Part model, mm, in its own coordinate system. A direction names the side the tool comes from. Round coordinates to 2 decimals unless told otherwise and drop trailing zeros. Write each loop counter-clockwise with the first axis right and the second up, starting at its lowest first coordinate (ties: lowest second). Pieces come first, ordered by that corner, then holes.
Autodesk Inventor part; units mm, degrees
ref_plane "YZ Plane" through (0, 0, 0) normal (1, 0, 0) x (0, 1, 0)
ref_plane "XZ Plane" through (0, 0, 0) normal (0, 1, 0) x (-1, 0, 0)
ref_plane "XY Plane" through (0, 0, 0) normal (0, 0, 1) x (1, 0, 0)
sketch "Esboço1" plane through (0, 0, 0) normal (0, 1, 0) x (-1, 0, 0)
  line L0 (5, 0) -> (70, 0)
  line L1 (75, -5) -> (75, -70)
  line L2 (70, -75) -> (5, -75)
  line L3 (0, -70) -> (0, -5)
  arc A0 (70, -75) -> (75, -70) centre (70, -70) ccw
  arc A1 (0, -70) -> (5, -75) centre (5, -70) ccw
  arc A2 (75, -5) -> (70, 0) centre (70, -5) ccw
  arc A3 (5, 0) -> (0, -5) centre (5, -5) ccw
  point P0 (0, 0)
  point P1 (75, -75)
  point P2 (75, 0)
  point P3 (0, -75)
  dimension "d0" = 75
  dimension "d1" = 75
  dimension "d2" = 5
extrude "Extrusão1" add sketch "Esboço1" along normal blind 5
sketch "Esboço2" plane through (0, 5, 0) normal (0, 1, 0) x (1, 0, 0)
  line L0 (0, 75) -> (-13, 75)
  line L1 (-75, 75) -> (-62, 75)
  line L2 (-75, 0) -> (-62, 0)
  line L3 (-70, 0) -> (-5, 0)
  line L4 (0, 0) -> (-13, 0)
  line L5 (-13, 75) -> (-13, 72.5)
  line L6 (-62, 75) -> (-62, 72.5)
  line L7 (-62, 0) -> (-62, 2.5)
  line L8 (-13, 0) -> (-13, 2.5)
  circle A0 centre (-62, 72.5) radius 1.25
  circle A1 centre (-13, 72.5) radius 1.25
  circle A2 centre (-62, 2.5) radius 1.25
  circle A3 centre (-13, 2.5) radius 1.25
  dimension "d5" = 13
  dimension "d6" = 2.5
  dimension "d7" = 2.5
  dimension "d8" = 2.5
  dimension "d9" = 2.5
  dimension "d10" = 2.5
  dimension "d11" = 2.5
extrude "Extrusão2" cut sketch "Esboço2" against normal through all
sketch "Esboço3" plane through (0, 0, 0) normal (0, -1, 0) x (1, 0, 0)
  line L0 (-5, -75) -> (-70, -75)
  line L1 (-5, -75) -> (-5, -70)
  line L2 (-5, -70) -> (-70, -70)
  line L3 (-70, -70) -> (-70, -5)
  line L4 (-70, -5) -> (-5, -5)
  line L5 (-5, -5) -> (-5, -70)
  point P0 (0, 0)
  dimension "d14" = 5
  dimension "d15" = 65
  dimension "d16" = 65
extrude "Extrusão3" cut sketch "Esboço3" against normal blind 2.5
sketch "Esboço4" plane through (0, 5, 0) normal (0, 1, 0) x (1, 0, 0)
  line L0 (-5, 70) -> (-70, 70)
  line L1 (-70, 70) -> (-65, 70)
  line L2 (-70, 70) -> (-70, 65)
  line L3 (-70, 65) -> (-65, 70)
  line L4 (-70, 5) -> (-5, 5)
  line L5 (-5, 5) -> (-5, 10)
  line L6 (-5, 5) -> (-5, 70)
  line L7 (-5, 5) -> (-10, 5)
  line L8 (-10, 5) -> (-5, 10)
  line L9 (-70, 65) -> (-70, 55)
  line L10 (-70, 70) -> (-70, 5)
  line L11 (-70, 55) -> (-67.5, 55)
  line L12 (-65, 70) -> (-55, 70)
  line L13 (-55, 70) -> (-55, 67.5)
  line L14 (-55, 67.5) -> (-63.9645, 67.5)
  line L15 (-65, 70) -> (-55, 70)
  line L16 (-70, 65) -> (-70, 55)
  line L17 (-67.5, 65) -> (-65, 67.5)
  line L18 (-67.5, 65) -> (-67.5, 55)
  line L19 (-65, 67.5) -> (-63.9645, 67.5)
  point P0 (0, 0)
sketch "Esboço5" plane through (0, 5, 0) normal (0, 1, 0) x (1, 0, 0)
  line L0 (-5, 5) -> (-5, 70)
  line L1 (-5, 10) -> (-5, 20)
  line L2 (-5, 20) -> (-7.5, 20)
  line L3 (-70, 5) -> (-5, 5)
  line L4 (-10, 5) -> (-20, 5)
  line L5 (-20, 5) -> (-20, 7.5)
  line L6 (-7.5, 10) -> (-10, 7.5)
  line L7 (-7.5, 20) -> (-7.5, 10)
  line L8 (-20, 7.5) -> (-10, 7.5)
  line L9 (-5, 20) -> (-5, 10)
  line L10 (-20, 5) -> (-10, 5)
  line L11 (-10, 5) -> (-5, 10)
  point P0 (0, 0)
  dimension "d23" = 2.5
  dimension "d24" = 10
  dimension "d25" = 2.5
extrude "Extrusão4" cut sketch "Esboço5" against normal through all contours L11 L3 L5 L8 L6 L7 L2 L0
extrude "Extrusão5" cut sketch "Esboço4" against normal through all contours L13 L14 L19 L17 L18 L11 L9 L3 L0
sketch "Esboço6" plane through (0, 5, 0) normal (0, 1, 0) x (1, 0, 0)
  line L0 (-70, 70) -> (-70, 5)
  line L1 (-5, 5) -> (-5, 70)
  line L2 (-70, 70) -> (-5, 70)
  line L3 (-5, 70) -> (-5, 5)
  line L4 (-5, 5) -> (-70, 5)
  line L5 (-70, 5) -> (-70, 70)
  arc A0 (0, 70) -> (-5, 75) centre (-5, 70) ccw
  line L6 (-5, 75) -> (0, 75)
  line L7 (0, 75) -> (0, 0)
  line L8 (0, 0) -> (-5, 0)
  line L9 (-5, 0) -> (-5, 75)
  line L10 (-75, 75) -> (0, 75)
  line L11 (0, 75) -> (0, 70)
  line L12 (0, 70) -> (-75, 70)
  line L13 (-75, 70) -> (-75, 75)
  line L14 (0, 0) -> (-75, 0)
  line L15 (-75, 0) -> (-75, 5)
  line L16 (-75, 5) -> (0, 5)
  line L17 (0, 5) -> (0, 0)
  line L18 (-75, 0) -> (-70, 0)
  line L19 (-70, 0) -> (-70, 75)
  line L20 (-70, 75) -> (-75, 75)
  line L21 (-75, 75) -> (-75, 0)
extrude "Extrusão6" cut sketch "Esboço6" against normal blind 1 contours L19 L10 L9 L2 | L0 L16 L21 L12 | L12 L13 L10 L19 | L19 L14 L15 L16 | L4 L9 L14 L19 | L12 L7 L16 L1 | L9 A0 L12 | L16 L7 L8 L9 | L6 L7 A0
thread "Rosca1"
thread "Rosca2"
thread "Rosca3"
thread "Rosca4"
properties part number "Tampa"
Q1. Cut at A-A on z = -17.5. Write the cut outline in (x, y).
Values follow:
outline: (-75, 0) - (-70, 0) - (-70, 2.5) - (-7.5, 2.5) - (-7.5, 5) - (-70, 5) - (-70, 4) - (-75, 4) - close; (-5, 0) - (0, 0) - (0, 4) - (-5, 4) - close
Q2. Drop flat-ended pins along their axis: pin 1 (3 mm diameter, centred on x = -13, z = -72.5, fed in from +Y); pin 2 (2.5 mm diameter, centred on x = -66.5, z = -68, fed in from -Y); pin 3 (0.5 mm diameter, centred on y = 4.5, z = -67.5, fed in from -X); pin 4 (2 mm diameter, centred on x = -62, z = -72.5, fed in from +Y). Give the stop position or say it passes through.
Values follow:
pin 1: stops at y = 4
pin 2: stops at y = 2.5
pin 3: stops at x = -70
pin 4: passes through
Q3. Wall check: L1, parallel to Z at x = -13, y = 2.45; L2, parallel to Z at x = -13, y = 2.95; L3, parallel to X at y = 2.05, z = -72.5. Give the ranges that are in metal, low to high.
Values follow:
L1: z = -75 to -73.75, -71.25 to -70, -5 to -3.75, -1.25 to 0
L2: z = -75 to -73.75, -71.25 to -7.5, -5 to -3.75, -1.25 to 0
L3: x = -74.33 to -63.25, -60.75 to -14.25, -11.75 to -0.67
Q4. Cut at D-D on z = -25.5. Write the cut outline in (x, y), plus the area to 4 significant figures.
Values follow:
outline: (-75, 0) - (-70, 0) - (-70, 2.5) - (-5, 2.5) - (-5, 0) - (0, 0) - (0, 4) - (-5, 4) - (-5, 5) - (-70, 5) - (-70, 4) - (-75, 4) - close
area: 202.5 mm2
Q5. Cut at C-C on y = 1.45. Write the cut outline in (x, z), plus the area to 3 significant figures.
Values follow:
outline: (-75, -70) arc R5 ccw to (-70, -75) - (-5, -75) arc R5 ccw to (0, -70) - (0, -5) arc R5 ccw to (-5, 0) - (-70, 0) arc R5 ccw to (-75, -5) - close; hole (-70, -70) - (-5, -70) - (-5, -5) - (-70, -5) - close; hole circle Ø2.5 at (-62, -72.5); hole circle Ø2.5 at (-62, -2.5); hole circle Ø2.5 at (-13, -72.5); hole circle Ø2.5 at (-13, -2.5)
area: 1,360 mm2
Q6. Which spindle directions (+Z, -Z, +X, -X, +Y, -Y) get a long thin tool onto all of the face, cutting with end or side? Do faces 4 (the flat face through (-66.3, 3.8, -66.2)), 5 (the flat face through (-69, 2.5, -69)), 6 (the flat face through (-37, 2, 0)). Say none if no direction does.
Values follow:
face 4: +Y, -Y
face 5: -Y
face 6: +Z, +X, -X, +Y, -Y
Q7. Mould opens along Z. For faces 1 (the flat face through (-20, 4, -6)), 2 (the cylindrical face through (-73, 2, -1)), 3 (the flat face through (-75, 2, -37)) say: +Z half, -Z half, draft (parallel to the pull), parting line (faces both ways), or undercut.
Values follow:
face 1: undercut
face 2: +Z half
face 3: draft
Q8. Cut at B-B on x = -62. Write the cut outline in (y, z).
Values follow:
outline: (0, -75) - (4, -75) - (4, -73.75) - (0, -73.75) - close; (0, -71.25) - (4, -71.25) - (4, -70) - (0, -70) - close; (0, -5) - (2.5, -5) - (2.5, -67.5) - (5, -67.5) - (5, -5) - (4, -5) - (4, -3.75) - (0, -3.75) - close; (0, -1.25) - (4, -1.25) - (4, 0) - (0, 0) - close
